from build123d import *

# Parameters (mm, degrees)
RESSALTO_EXTRUS_O1_DEPTH = 1
FILETE1_R                = 5
FILETE2_R                = 6.5
FILETE3_R                = 8
FILETE4_R                = 1.5
FILETE5_R                = 2.5
FILETE6_R                = 2.5
FILETE7_R                = 2.5
FILETE9_R                = 5
FILETE10_R               = 2.5
FILETE11_R               = 2.5
ESBO_O2_R                = 2.65
ESBO_O2_R_2              = 3.15
CORTE_EXTRUS_O1_DEPTH    = 1
ESBO_O3_R                = 76.25
CORTE_EXTRUS_O2_DEPTH    = 1


with BuildPart() as part:
    # Esboço1 → Ressalto-extrusão1 (new body)
    with BuildSketch(Plane.XY):
        Polygon((-28.900998415, -44.564212679), (-50.493725783, -39.180541088), (-50.493725783, -7.064212679), (-41.23351444, 21.435787321), (-32.705131271, 21.435787321), (-29.613232907, 43.435787321), (18.886767093, 43.435787321), (18.886767093, 27.435787321), (-5.993725783, 25.695973775), (-5.993725783, 22.695973775), (20.558362115, 19.435787321), (29.006274217, -6.564212679), (29.006274217, -38.437470915), (4.433255164, -44.564212679), align=None)
    extrude(amount=RESSALTO_EXTRUS_O1_DEPTH)

    # Filete1
    filete1_edges = [part.edges().sort_by_distance(p)[0] for p in [
        (-32.705131271, 21.435787321, 0.5),
    ]]
    fillet(filete1_edges, radius=FILETE1_R)

    # Filete2
    filete2_edges = [part.edges().sort_by_distance(p)[0] for p in [
        (-29.613232907, 43.435787321, 0.5),
    ]]
    fillet(filete2_edges, radius=FILETE2_R)

    # Filete3
    filete3_edges = [part.edges().sort_by_distance(p)[0] for p in [
        (18.886767093, 43.435787321, 0.5),
        (18.886767093, 27.435787321, 0.5),
    ]]
    fillet(filete3_edges, radius=FILETE3_R)

    # Filete4
    filete4_edges = [part.edges().sort_by_distance(p)[0] for p in [
        (-5.993725783, 25.695973775, 0.5),
        (-5.993725783, 22.695973775, 0.5),
    ]]
    fillet(filete4_edges, radius=FILETE4_R)

    # Filete5
    filete5_edges = [part.edges().sort_by_distance(p)[0] for p in [
        (20.558362115, 19.435787321, 0.5),
    ]]
    fillet(filete5_edges, radius=FILETE5_R)

    # Filete6
    filete6_edges = [part.edges().sort_by_distance(p)[0] for p in [
        (29.006274217, -6.564212679, 0.5),
    ]]
    fillet(filete6_edges, radius=FILETE6_R)

    # Filete7
    filete7_edges = [part.edges().sort_by_distance(p)[0] for p in [
        (29.006274217, -38.437470915, 0.5),
    ]]
    fillet(filete7_edges, radius=FILETE7_R)

    # Filete9
    filete9_edges = [part.edges().sort_by_distance(p)[0] for p in [
        (-28.900998415, -44.564212679, 0.5),
        (4.433255164, -44.564212679, 0.5),
    ]]
    fillet(filete9_edges, radius=FILETE9_R)

    # Filete10
    filete10_edges = [part.edges().sort_by_distance(p)[0] for p in [
        (-50.493725783, -39.180541088, 0.5),
        (-50.493725783, -7.064212679, 0.5),
    ]]
    fillet(filete10_edges, radius=FILETE10_R)

    # Filete11
    filete11_edges = [part.edges().sort_by_distance(p)[0] for p in [
        (-41.23351444, 21.435787321, 0.5),
    ]]
    fillet(filete11_edges, radius=FILETE11_R)

    # Esboço2 → Corte-extrusão1 (cut)
    with BuildSketch(Plane.XY.offset(1)):
        with Locations((-24.993725783, -26.564212679)):
            Circle(ESBO_O2_R)
        with Locations((11.006274217, -26.564212679)):
            Circle(ESBO_O2_R)
        with Locations((-24.993725783, 14.435787321)):
            Circle(ESBO_O2_R)
        with Locations((11.006274217, 14.435787321)):
            Circle(ESBO_O2_R)
        with Locations((-23.243725783, 36.435787321)):
            Circle(ESBO_O2_R_2)
        with Locations((9.256274217, 36.435787321)):
            Circle(ESBO_O2_R_2)
    extrude(amount=-CORTE_EXTRUS_O1_DEPTH, mode=Mode.SUBTRACT)

    # Esboço3 → Corte-extrusão2 (cut)
    with BuildSketch(Plane.XY.offset(1)):
        with Locations((-6.993725783, 117.935787321)):
            Circle(ESBO_O3_R)
    extrude(amount=-CORTE_EXTRUS_O2_DEPTH, mode=Mode.SUBTRACT)


solid = part.part
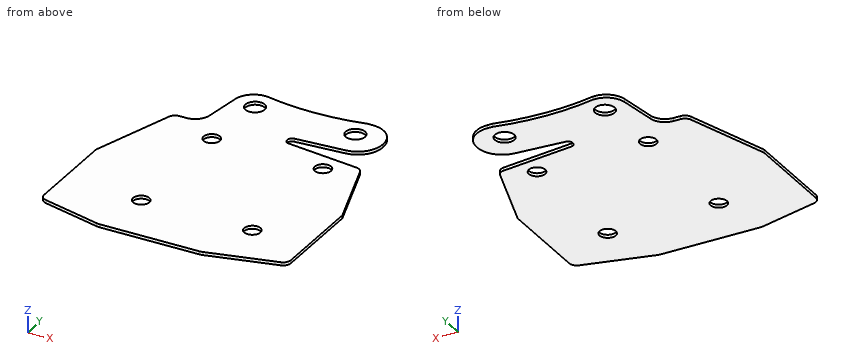
CAD build for the part. Positions are in the model's coordinates, mm. Round coordinates to 2 decimals unless told otherwise and drop trailing zeros. Loops run counter-clockwise (first coordinate to the right, second up) from the corner with the lowest first, then second, coordinate; pieces in that order, holes last. Notation, with made-up numbers: M 49,28.5 L 67,28.5 A16 cw 67,49.5 Z; hole C 3.5,-31 d6. An arc over 180 degrees is marked long. One line per question, with ' | ' between items. Start each with the question number.
Item 1: Wall check: line 1 (X direction, y = 37, z = 0.75); line 2 (Y direction, x = -1, z = 0.2); line 3 (Y direction, x = 13, z = 0.5). Give the ranges that are in metal, low to high.
Item 2: Cut at B-B, the plane z = 0.15. State how many separate pieces and enclosed holes the cut face has, plus the area to 3 significant figures.
Item 3: Cut at C-C, the plane y = 10. Write the cut outline in (x, z), plus the area to 3 significant figures.
Item 4: Cut at A-A, the plane x = -3. Write the cut outline in (y, z), plus the area to 3 significant figures.
Item 5: Cut at D-D, the plane x = -43.5. Write the cut outline in (y, z), plus the area to 3 significant figures.
Responses:
1) line 1: x = -30.52 to -26.34, -20.14 to 6.16, 12.36 to 18.73 | line 2: y = -44.56 to 22.08, 26.05 to 41.92 | line 3: y = -42.43 to -28.31, -24.82 to 12.69, 16.18 to 20.36, 27.18 to 43.15
2) separate pieces: 1 | enclosed holes: 6 | area: 5,600 mm²
3) outline: M -44.95,0 L 23.62,0 L 23.62,1 L -44.95,1 Z | area: 68.6 mm²
4) outline: M -44.56,0 L 22.33,0 L 22.33,1 L -44.56,1 Z; M 25.91,0 L 41.79,0 L 41.79,1 L 25.91,1 Z | area: 82.8 mm²
5) outline: M -40.92,0 L 14.46,0 L 14.46,1 L -40.92,1 Z | area: 55.4 mm²
